Part model, mm, in its own coordinate system. Face numbers are marked on the shaded views. Round coordinates to 2 decimals unless told otherwise and drop trailing zeros. Write each loop counter-clockwise with the first axis right and the second up, starting at its lowest first coordinate (ties: lowest second). Pieces come first, ordered by that corner, then holes.
1) Flat gauge pins, fed straight in: pin 1 (4 mm diameter, centred on y = 0, z = -7.5, fed in from +X); pin 2 (6.5 mm diameter, centred on x = 8.75, y = 0, fed in from -Z); pin 3 (4 mm diameter, centred on y = -5, z = -11, fed in from +X); pin 4 (3.5 mm diameter, centred on x = 9, y = -8.5, fed in from -Z). Where does each tip first touch, or does it go through?
2) Pull direction Y, two halves, no side cores. Call the marked faces 1, 2, 3 and 4: +Y half, -Y half, draft (parallel to the pull), parting line (faces both ways), or undercut.
3) Saw through at C-C on y = 1.25. Write the cut outline in (x, z), and give its area (3 significant figures).
4) Saw through at B-B on x = 8.75. Write the cut outline in (y, z), and give its area (3 significant figures).
5) Saw through at A-A on z = -7.5. Write the cut outline in (x, y), and give its area (3 significant figures).
6) Drill centre lines: L1, parallel to Y at x = 8.75, z = 1.45; L2, parallel to X at y = 6.5, z = -1.5; L3, parallel to Y at x = -12, z = -6.5. Where is each one in solid material? Low to high.
7) Saw through at D-D on y = 7. Write the cut outline in (x, z).
```python
from build123d import *

# Parameters (mm, degrees)
SKETCH1_W           = 32.5
SKETCH1_H           = 20
BOSS_EXTRUDE1_DEPTH = 5
SKETCH2_W           = 5
SKETCH2_H           = 20
BOSS_EXTRUDE2_DEPTH = 15
SKETCH3_R           = 2.5
CUT_EXTRUDE1_DEPTH  = 15
SKETCH4_R           = 2.5
CUT_EXTRUDE2_DEPTH  = 15
SKETCH5_W           = 5
SKETCH5_H           = 4
BOSS_EXTRUDE3_DEPTH = 3
FILLET1_R           = 1
FILLET2_R           = 2
CUT_EXTRUDE3_DEPTH  = 2.2


with BuildPart() as part:
    # Sketch1 → Boss-Extrude1 (new body)
    with BuildSketch(Plane.XY):
        Rectangle(SKETCH1_W, SKETCH1_H)
    extrude(amount=BOSS_EXTRUDE1_DEPTH)

    # Sketch2 → Boss-Extrude2 (add)
    with BuildSketch(Plane(origin=(0, 0, 0), x_dir=(-1, 0, 0), z_dir=(0, 0, -1))):
        with Locations((13.75, 0)):
            Rectangle(SKETCH2_W, SKETCH2_H)
    extrude(amount=BOSS_EXTRUDE2_DEPTH)

    # Sketch3 → Cut-Extrude1 (cut)
    with BuildSketch(Plane(origin=(-11.25, 0, 0), x_dir=(0, 0, -1), z_dir=(1, 0, 0))):
        with Locations(Location((7.5, 0, 0), (0, 0, 90))):
            Circle(SKETCH3_R)
    extrude(amount=-CUT_EXTRUDE1_DEPTH, mode=Mode.SUBTRACT)

    # Sketch4 → Cut-Extrude2 (cut)
    with BuildSketch(Plane.XY.offset(5)):
        with Locations((8.75, 0)):
            Circle(SKETCH4_R)
    extrude(amount=-CUT_EXTRUDE2_DEPTH, mode=Mode.SUBTRACT)

    # Sketch5 → Boss-Extrude3 (add)
    with BuildSketch(Plane(origin=(0, 0, 0), x_dir=(-1, 0, 0), z_dir=(0, 0, -1))):
        with Locations((-8.75, 8)):
            Rectangle(SKETCH5_W, SKETCH5_H)
        with Locations((-8.75, -8)):
            Rectangle(SKETCH5_W, SKETCH5_H)
    extrude(amount=BOSS_EXTRUDE3_DEPTH)

    # Fillet1
    fillet1_edges = [part.edges().sort_by_distance(p)[0] for p in [
        (11.25, 8, -3),
        (6.25, 8, -3),
        (6.25, -8, -3),
        (11.25, -8, -3),
    ]]
    fillet(fillet1_edges, radius=FILLET1_R)

    # Fillet2
    fillet2_edges = [part.edges().sort_by_distance(p)[0] for p in [
        (-13.75, 10, -15),
        (-13.75, -10, -15),
        (16.25, 10, 2.5),
        (16.25, -10, 2.5),
    ]]
    fillet(fillet2_edges, radius=FILLET2_R)

    # Sketch6 → Cut-Extrude3 (cut)
    with BuildSketch(Plane(origin=(-11.25, 0, 0), x_dir=(0, 0, -1), z_dir=(1, 0, 0))):
        Polygon((3.227608008, 0), (5.363804004, -3.7), (9.636195996, -3.7), (11.772391992, 0), (9.636195996, 3.7), (5.363804004, 3.7), align=None)
    extrude(amount=-CUT_EXTRUDE3_DEPTH, mode=Mode.SUBTRACT)


solid = part.part
```
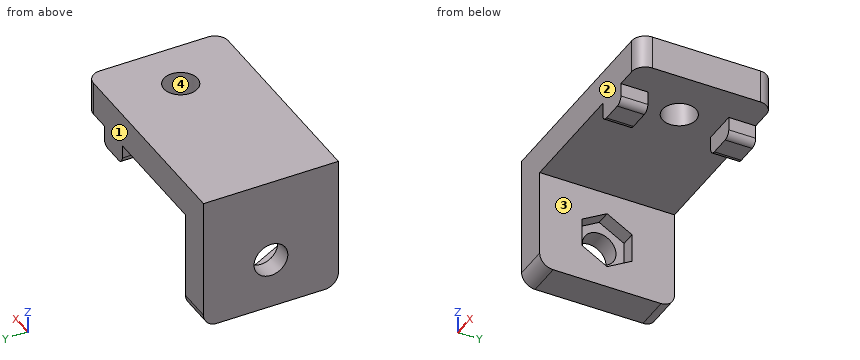
Completed:
1. pin 1: passes through
1. pin 2: stops at z = 0
1. pin 3: stops at x = -11.25
1. pin 4: stops at z = -3
2. face 1: +Y half
2. face 2: -Y half
2. face 3: draft
2. face 4: undercut
3. outline: (-16.25, -15) - (-11.25, -15) - (-11.25, -11.05) - (-13.45, -11.05) - (-13.45, -9.67) - (-16.25, -9.67) - close; (-16.25, -5.33) - (-13.45, -5.33) - (-13.45, -3.95) - (-11.25, -3.95) - (-11.25, 0) - (6.58, 0) - (6.58, 5) - (-16.25, 5) - close; (10.92, 0) - (16.25, 0) - (16.25, 5) - (10.92, 5) - close
3. area: 188 mm2
4. outline: (-10, -3) - (-6, -3) - (-6, 0) - (-2.5, 0) - (-2.5, 5) - (-10, 5) - close; (2.5, 0) - (6, 0) - (6, -3) - (10, -3) - (10, 5) - (2.5, 5) - close
4. area: 99.0 mm2
5. outline: (-16.25, -10) - (-11.25, -10) - (-11.25, -3.7) - (-13.45, -3.7) - (-13.45, -2.5) - (-16.25, -2.5) - close; (-16.25, 2.5) - (-13.45, 2.5) - (-13.45, 3.7) - (-11.25, 3.7) - (-11.25, 10) - (-16.25, 10) - close
5. area: 69.7 mm2
6. L1: y = -10 to -2.5, 2.5 to 10
6. L2: x = -16.25 to -11.25, 6.25 to 11.25
6. L3: y = -10 to -3.7, 3.7 to 10
7. outline: (-16.25, -15) - (-11.25, -15) - (-11.25, 0) - (6.25, 0) - (6.25, -2) arc R1 ccw to (7.25, -3) - (10.25, -3) arc R1 ccw to (11.25, -2) - (11.25, 0) - (16.25, 0) - (16.25, 5) - (-16.25, 5) - close
